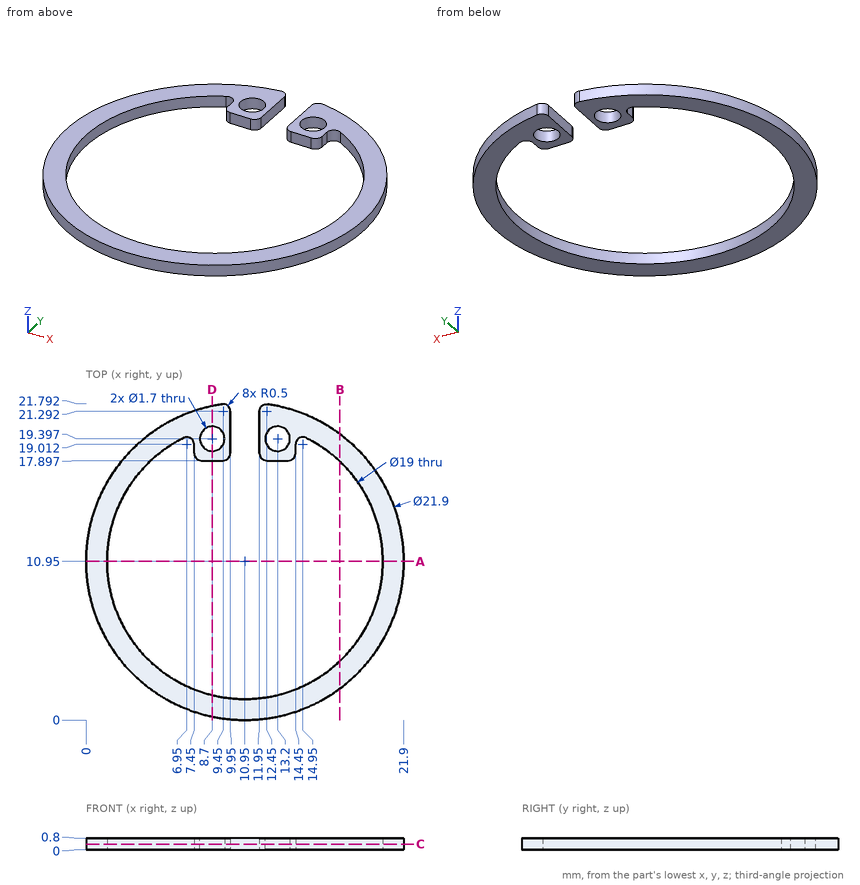
Could you check a few things on this drawing? It's one solid part, dimensions in mm from its lowest x, y, z. Give positions to 0.01 mm unless a question says otherwise; leave off trailing zeros. Loops run counter-clockwise (first coordinate to the right, second up) from the corner with the lowest first, then second, coordinate; pieces in that order, holes last. Notation, with made-up numbers: M 80,-13.5 L 109,-13.5 A21 cw 109,-7.5 Z; hole C 53.25,75 d7. An arc over 180 degrees is marked long. One line per question, with ' | ' between items. Start each with the question number.
Q1. If we section it at B-B (x = 17.5): Please give me the cut outline in (y, z) (1 decimal).
Q2. If we section it at C-C (z = 0.4): Please give me the cut outline in (x, y).
Q3. If we section it at A-A (y = 10.95): Please give me the cut outline in (x, z), plus the area to 3 significant figures.
Q4. If we section it at D-D (x = 8.7): Please give me the cut outline in (y, z).
Q5. If I drill on line 1 (Y direction, x = 8.7, z = 0.55); line 2 (Y direction, x = 9.75, z = 0.35) (1 decimal); line 3 (Y direction, x = 3, z = 0.6), over which ranges is the centre line in solid material (lowest first)? Write a range as from..to.
Computed:
1) outline: M 2.2,0 L 4.1,0 L 4.1,0.8 L 2.2,0.8 Z; M 17.8,0 L 19.7,0 L 19.7,0.8 L 17.8,0.8 Z
2) outline: M 6.73,19.46 A0.5 cw 7.45,19.01 L 7.45,18.4 A0.5 ccw 7.95,17.9 L 9.45,17.9 A0.5 ccw 9.95,18.4 L 9.95,21.29 A0.5 ccw 9.38,21.79 A10.95 ccw long 12.52,21.79 A0.5 ccw 11.95,21.29 L 11.95,18.4 A0.5 ccw 12.45,17.9 L 13.95,17.9 A0.5 ccw 14.45,18.4 L 14.45,19.01 A0.5 cw 15.17,19.46 A9.5 cw long Z; hole C 8.7,19.4 d1.7; hole C 13.2,19.4 d1.7
3) outline: M 0,0 L 1.45,0 L 1.45,0.8 L 0,0.8 Z; M 20.45,0 L 21.9,0 L 21.9,0.8 L 20.45,0.8 Z | area: 2.32 mm²
4) outline: M 0.23,0 L 1.72,0 L 1.72,0.8 L 0.23,0.8 Z; M 17.9,0 L 18.55,0 L 18.55,0.8 L 17.9,0.8 Z; M 20.25,0 L 21.67,0 L 21.67,0.8 L 20.25,0.8 Z
5) line 1: y = 0.23..1.72, 17.9..18.55, 20.25..21.67 | line 2: y = 0.1..1.5, 18..21.7 | line 3: y = 3.42..5.75, 16.15..18.48
